Work out the finished part from the listing and answer in its coordinate system (mm). A direction names the side the tool comes from. Round coordinates to 2 decimals unless told otherwise and drop trailing zeros. Order: outer loops, then holes, each group sorted by start corner. A loop starts at its lowest first (then second) coordinate and runs counter-clockwise, first axis right, second up. Notation, with made-up numbers: (41, -29.75) -> (49, -29.75) arc R27 ccw to (49, -3.75) -> close; hole circle Ø6 at (-21, -17). An arc over 180 degrees is marked (long way). Use a Markdown table: item, result. Add a question column.
Item 1: A cutting plane is placed at A-A, the plane x = 0. Determine the outline of the cut face in (y, z).
Item 2: A cutting plane is placed at D-D, the plane y = -15. Determine the outline of the cut face in (x, z).
Item 3: Find the intervals of material crossed by L1, parallel to X at y = -19.5, z = 30.5; L2, parallel to Y at x = -46, z = 33.5; L3, parallel to X at y = 1, z = 20.5, in increasing order. Write a range as [from, to].
Item 4: A tool of negligible diameter and unlimited length cuts with its end or side. For faces 4 (the flat face through (-38, 1.891, 19)), 5 (the flat face through (23, -11, 0)), from which of +Z, -Z, +X, -X, +Y, -Y can it reach the whole face along a straight path? Write none if from no direction.
Item 5: Flat-ended cylindrical pins translate along their axes: P1, Ø7.5, axis at x = 42.5, z = 18.5, coming from the -Y side; P2, Ø3, axis at y = 31, z = 29, coming from the +X side; P3, Ø8, axis at y = 41.5, z = 8.5, coming from the -X side; P4, Ø1, axis at x = -7, y = -20, coming from the +Z side. Find the tip coordinate at first contact, or state that the pin passes through.
Item 6: For a pull along Y with two mould halves and no side action, classify faces 1 (the flat face through (27, 0, 35)), 2 (the flat face through (-38, -1.891, 19)), 3 (the cylindrical face through (-6.9, 52.8, 17.3)) as +Y half, -Y half, draft (parallel to the pull), parting line (faces both ways), or undercut.
Item 7: A cutting plane is placed at B-B, the plane z = 44. Determine the outline of the cut face in (x, y), plus the area to 3 significant figures.
from build123d import *

# Parameters (mm, degrees)
F0_R     = 53.25
F1_DEPTH = 35
F2_DEPTH = 4
F3_DEPTH = 50


with BuildPart() as f1:
    # F0 (on Top) → F1 (new body)
    with BuildSketch(Plane.XY):
        Circle(F0_R)
        with BuildLine():
            ThreePointArc((-50.4645979232, 1.8905968509), (0, 50.5), (50.4645979232, 1.8905968509))
            ThreePointArc((50.4645979232, 1.8905968509), (50.4911487051, 0.94546414), (50.5, 0))
            ThreePointArc((50.5, 0), (50.4911487051, -0.94546414), (50.4645979232, -1.8905968509))
            ThreePointArc((50.4645979232, -1.8905968509), (0, -50.5), (-50.4645979232, -1.8905968509))
            ThreePointArc((-50.4645979232, -1.8905968509), (-50.5, 0), (-50.4645979232, 1.8905968509))
        make_face(mode=Mode.SUBTRACT)
        with BuildLine():
            ThreePointArc((-25.4298180007, -1.8905968509), (-25.5, 0), (-25.4298180007, 1.8905968509))
            Line((-25.4298180007, 1.8905968509), (-50.4645979232, 1.8905968509))
            ThreePointArc((-50.4645979232, 1.8905968509), (-50.5, 0), (-50.4645979232, -1.8905968509))
            Line((-50.4645979232, -1.8905968509), (-25.4298180007, -1.8905968509))
        make_face()
        with BuildLine():
            Line((50.4645979232, 1.8905968509), (25.4298180007, 1.8905968509))
            ThreePointArc((25.4298180007, 1.8905968509), (25.4824484598, 0.9459495184), (25.5, 0))
            ThreePointArc((25.5, 0), (25.4824484598, -0.9459495184), (25.4298180007, -1.8905968509))
            Line((25.4298180007, -1.8905968509), (50.4645979232, -1.8905968509))
            ThreePointArc((50.4645979232, -1.8905968509), (50.4911487051, -0.94546414), (50.5, 0))
            ThreePointArc((50.5, 0), (50.4911487051, 0.94546414), (50.4645979232, 1.8905968509))
        make_face()
    extrude(amount=F1_DEPTH)

    # F0 (on Top) → F2 (join)
    with BuildSketch(Plane.XY):
        with BuildLine():
            ThreePointArc((-25.4298180007, 1.8905968509), (0, 25.5), (25.4298180007, 1.8905968509))
            Line((25.4298180007, 1.8905968509), (50.4645979232, 1.8905968509))
            ThreePointArc((50.4645979232, 1.8905968509), (0, 50.5), (-50.4645979232, 1.8905968509))
            Line((-50.4645979232, 1.8905968509), (-25.4298180007, 1.8905968509))
        make_face()
        with BuildLine():
            Line((50.4645979232, -1.8905968509), (25.4298180007, -1.8905968509))
            ThreePointArc((25.4298180007, -1.8905968509), (0, -25.5), (-25.4298180007, -1.8905968509))
            Line((-25.4298180007, -1.8905968509), (-50.4645979232, -1.8905968509))
            ThreePointArc((-50.4645979232, -1.8905968509), (0, -50.5), (50.4645979232, -1.8905968509))
        make_face()
    extrude(amount=F2_DEPTH)

    # F0 (on Top) → F3 (join)
    with BuildSketch(Plane.XY):
        with BuildLine():
            ThreePointArc((-22.9221648966, 1.8905968509), (0, 23), (22.9221648966, 1.8905968509))
            Line((22.9221648966, 1.8905968509), (25.4298180007, 1.8905968509))
            ThreePointArc((25.4298180007, 1.8905968509), (0, 25.5), (-25.4298180007, 1.8905968509))
            Line((-25.4298180007, 1.8905968509), (-22.9221648966, 1.8905968509))
        make_face()
        with BuildLine():
            Line((25.4298180007, -1.8905968509), (22.9221648966, -1.8905968509))
            ThreePointArc((22.9221648966, -1.8905968509), (0, -23), (-22.9221648966, -1.8905968509))
            Line((-22.9221648966, -1.8905968509), (-25.4298180007, -1.8905968509))
            ThreePointArc((-25.4298180007, -1.8905968509), (0, -25.5), (25.4298180007, -1.8905968509))
        make_face()
        with BuildLine():
            ThreePointArc((-22.9221648966, -1.8905968509), (-23, 0), (-22.9221648966, 1.8905968509))
            Line((-22.9221648966, 1.8905968509), (-25.4298180007, 1.8905968509))
            ThreePointArc((-25.4298180007, 1.8905968509), (-25.5, 0), (-25.4298180007, -1.8905968509))
            Line((-25.4298180007, -1.8905968509), (-22.9221648966, -1.8905968509))
        make_face()
        with BuildLine():
            ThreePointArc((22.9221648966, 1.8905968509), (22.9805329858, 0.9460991962), (23, 0))
            ThreePointArc((23, 0), (22.9805329858, -0.9460991962), (22.9221648966, -1.8905968509))
            Line((22.9221648966, -1.8905968509), (25.4298180007, -1.8905968509))
            ThreePointArc((25.4298180007, -1.8905968509), (25.4824484598, -0.9459495184), (25.5, 0))
            ThreePointArc((25.5, 0), (25.4824484598, 0.9459495184), (25.4298180007, 1.8905968509))
            Line((25.4298180007, 1.8905968509), (22.9221648966, 1.8905968509))
        make_face()
    extrude(amount=F3_DEPTH)


solid = f1.part
Reported:
| question | item | result |
|---|---|---|
| 1 | outline | (-53.25, 0) -> (-23, 0) -> (-23, 50) -> (-25.5, 50) -> (-25.5, 4) -> (-50.5, 4) -> (-50.5, 35) -> (-53.25, 35) -> close; (23, 0) -> (53.25, 0) -> (53.25, 35) -> (50.5, 35) -> (50.5, 4) -> (25.5, 4) -> (25.5, 50) -> (23, 50) -> close |
| 2 | outline | (-51.09, 0) -> (-17.44, 0) -> (-17.44, 50) -> (-20.62, 50) -> (-20.62, 4) -> (-48.22, 4) -> (-48.22, 35) -> (-51.09, 35) -> close; (17.44, 0) -> (51.09, 0) -> (51.09, 35) -> (48.22, 35) -> (48.22, 4) -> (20.62, 4) -> (20.62, 50) -> (17.44, 50) -> close |
| 3 | L1 | [-49.55, -46.58], [-16.43, -12.2], [12.2, 16.43], [46.58, 49.55] |
| 3 | L2 | [-26.82, -20.84], [-1.89, 1.89], [20.84, 26.82] |
| 3 | L3 | [-53.24, -22.98], [22.98, 53.24] |
| 4 | face 4 | +Z |
| 4 | face 5 | -Z, +X, -X, +Y, -Y |
| 5 | P1 | y = -36.52 |
| 5 | P2 | x = 44.33 |
| 5 | P3 | x = -37.81 |
| 5 | P4 | through |
| 6 | face 1 | draft |
| 6 | face 2 | undercut |
| 6 | face 3 | parting line |
| 7 | outline | circle Ø51 at (0, 0); hole circle Ø46 at (0, 0) |
| 7 | area | 381 mm² |
